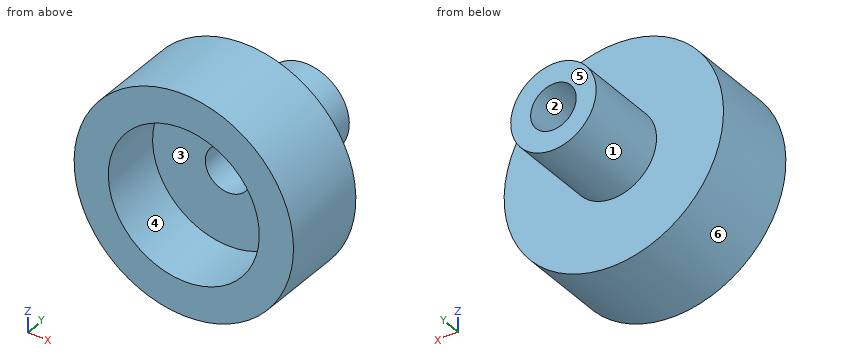
```python
from build123d import *

# Parameters (mm, degrees)
SKETCH1_R               = 3.85
BOSS_EXTRUDE1_DEPTH     = 3.1
SKETCH2_R               = 1.5
SKETCH2_R_2             = 0.8
BOSS_EXTRUDE2_DEPTH     = 3
CUT_EXTRUDE1_DEPTH      = 7.265381074
CUT_EXTRUDE1_DEPTH_BACK = 7.265381074
SKETCH3_R               = 0.8
SKETCH4_R               = 2.65
CUT_EXTRUDE2_DEPTH      = 2.2


with BuildPart() as part:
    # Sketch1 → Boss-Extrude1 (new body)
    with BuildSketch(Plane(origin=(0, 0, 0), x_dir=(1, 0, 0), z_dir=(0, 1, 0))):
        with Locations(Location((0, 0, 0), (0, 0, 90))):
            Circle(SKETCH1_R)
    extrude(amount=BOSS_EXTRUDE1_DEPTH)

    # Sketch2 → Boss-Extrude2 (add)
    with BuildSketch(Plane(origin=(0, 3.1, 0), x_dir=(1, 0, 0), z_dir=(0, 1, 0))):
        with Locations(Location((0, 0, 0), (0, 0, 270))):
            Circle(SKETCH2_R)
        with Locations(Location((0, 0, 0), (0, 0, 270))):
            Circle(SKETCH2_R_2, mode=Mode.SUBTRACT)
    extrude(amount=BOSS_EXTRUDE2_DEPTH)

    # Sketch3 → Cut-Extrude1 (cut, two sides: drawn at the far end of the back side and taken through both)
    with BuildSketch(Plane(origin=(0, 3.1, 0), x_dir=(1, 0, 0), z_dir=(0, 1, 0)).offset(-CUT_EXTRUDE1_DEPTH_BACK)):
        with Locations(Location((0, 0, 0), (0, 0, 270))):
            Circle(SKETCH3_R)
    extrude(amount=CUT_EXTRUDE1_DEPTH + CUT_EXTRUDE1_DEPTH_BACK, mode=Mode.SUBTRACT)

    # Sketch4 → Cut-Extrude2 (cut)
    with BuildSketch(Plane.XZ):
        with Locations(Location((0, 0, 0), (0, 0, 270))):
            Circle(SKETCH4_R)
    extrude(amount=-CUT_EXTRUDE2_DEPTH, mode=Mode.SUBTRACT)


solid = part.part
```
Geometry: final body of the model. Coordinates: model frame, mm. Face numbers are marked on the shaded views. A direction names the side the tool comes from. Round coordinates to 2 decimals unless told otherwise and drop trailing zeros. Write each loop counter-clockwise with the first axis right and the second up, starting at its lowest first coordinate (ties: lowest second). Pieces come first, ordered by that corner, then holes.
Item 1: Material intervals for L1, parallel to X at y = 0.95, z = 0; L2, parallel to X at y = 4, z = 0; L3, parallel to Y at x = 2.75, z = 2.5, sorted ascending.
Item 2: Section query B-B (x = 0). Return loops of the section in (y, z), plus the area to 3 significant figures.
Item 3: Section query D-D (z = 2.25). Return loops of the section in (x, y).
Item 4: Set-up query: the marked faces 1, 2 and 3. Return all of +Z, -Z, +X, -X, +Y, -Y with unobstructed straight access to the full face (end or side cutting, diameter ignored); none if empty.
Item 5: Section query C-C (y = 3). Return loops of the section in (x, z), plus the area to 3 significant figures.
Item 6: Mould query, pull axis X, two halves, no side actions, for the marked faces 4, 5 and 6. Classes: +X half, -X half, draft (parallel to the pull), parting line (faces both ways), or undercut.
Item 7: Pin query (flat end, axial travel): P1, Ø3, axis at x = 2, y = 3.5, coming from the +Z side; P2, Ø1, axis at x = -2.5, y = 1.5, coming from the +Z side; P3, Ø2, axis at y = 2.5, z = 1.5, coming from the -X side. Return the tip coordinate at first contact, or that it passes through.
Item 8: Section query A-A (z = 0). Return loops of the section in (x, y), plus the area to 3 significant figures.
Completed:
1. L1: x = -3.85 to -2.65, 2.65 to 3.85
1. L2: x = -1.5 to -0.8, 0.8 to 1.5
1. L3: y = 0 to 3.1
2. outline: (0, -3.85) - (3.1, -3.85) - (3.1, -1.5) - (6.1, -1.5) - (6.1, -0.8) - (2.2, -0.8) - (2.2, -2.65) - (0, -2.65) - close; (0, 2.65) - (2.2, 2.65) - (2.2, 0.8) - (6.1, 0.8) - (6.1, 1.5) - (3.1, 1.5) - (3.1, 3.85) - (0, 3.85) - close
2. area: 15.0 mm2
3. outline: (-3.12, 0) - (-1.4, 0) - (-1.4, 2.2) - (1.4, 2.2) - (1.4, 0) - (3.12, 0) - (3.12, 3.1) - (-3.12, 3.1) - close
4. face 1: +Y
4. face 2: +Y, -Y
4. face 3: -Y
5. outline: circle Ø7.7 at (0, 0); hole circle Ø1.6 at (0, 0)
5. area: 44.6 mm2
6. face 4: undercut
6. face 5: draft
6. face 6: parting line
7. P1: stops at z = 3.81
7. P2: stops at z = 3.29
7. P3: stops at x = -3.82
8. outline: (-3.85, 0) - (-2.65, 0) - (-2.65, 2.2) - (-0.8, 2.2) - (-0.8, 6.1) - (-1.5, 6.1) - (-1.5, 3.1) - (-3.85, 3.1) - close; (0.8, 2.2) - (2.65, 2.2) - (2.65, 0) - (3.85, 0) - (3.85, 3.1) - (1.5, 3.1) - (1.5, 6.1) - (0.8, 6.1) - close
8. area: 15.0 mm2
